Read the model definition and answer for the solid it produces. Units are mm, in the model's axes. Face numbers are marked on the shaded views. A direction names the side the tool comes from. Coordinates: 2 decimals unless noted, no trailing zeros. Order: outer loops, then holes, each group sorted by start corner. A loop starts at its lowest first (then second) coordinate and runs counter-clockwise, first axis right, second up.
from build123d import *

# Parameters (mm, degrees)
R_VOLUTION1_ANGLE  = 180
COQUE1_T           = -2
ESQUISSE2_W        = 60
ESQUISSE2_H        = 8
BOSS_EXTRU_1_DEPTH = 8
CHANFREIN1_SIZE    = 1


with BuildPart() as part:
    # Esquisse1 → Révolution1 (revolve)
    with BuildSketch(Plane.XY):
        with BuildLine():
            Line((-25, 0), (25, 0))
            ThreePointArc((25, 0), (0, 25), (-25, 0))
        make_face()
    revolve(axis=Axis((-25, 0, 0), (1, 0, 0)), revolution_arc=R_VOLUTION1_ANGLE)

    # Coque1
    coque1_openings = [part.faces().sort_by_distance(p)[0] for p in [
        (-25, 0, 0),
    ]]
    offset(amount=COQUE1_T, openings=coque1_openings)

    # Esquisse2 → Boss.-Extru.1 (add)
    with BuildSketch(Plane.XY):
        with Locations((52.649503306, 0)):
            Rectangle(ESQUISSE2_W, ESQUISSE2_H)
    extrude(amount=BOSS_EXTRU_1_DEPTH)

    # Chanfrein1
    chanfrein1_edges = [part.edges().sort_by_distance(p)[0] for p in [
        (82.649503306, -4, 4),
        (82.649503306, 4, 4),
    ]]
    chamfer(chanfrein1_edges, length=CHANFREIN1_SIZE)


solid = part.part
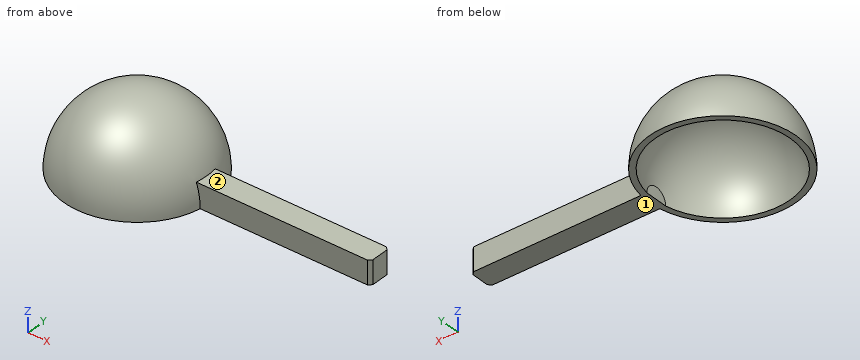
Q1. Which of the six approach directions +Z, -Z, +X, -X, +Y, -Y give full straight-line access (tool end or side, diameter ignored) to the marked faces 1 and 2?
Q2. Each of these flat-tipped pins is pushed along its axis until it touches: P1, Ø4, axis at x = 55.5, z = 2, coming from the +Y side; P2, Ø2, axis at y = 1.5, z = 3, coming from the -X side; P3, Ø12, axis at x = 15.5, y = -16.5, coming from the +Z side; P4, Ø8, axis at y = -1.5, z = 8.5, coming from the +X side. Where does it stop, or does it pass through?
Q3. Straight lines are drawn through the part: L1, parallel to Y at x = 16.5, z = 3; L2, parallel to X at y = -15, z = 9; L3, parallel to X at y = 17, z = 12.75. For each, find the intervals that lie inside material, in ascending order.
Q4. The part is cut by section B-B, the plane x = 32. Determine the outline of the cut face in (y, z), then the cut area to 3 significant figures.
Q5. The part is cut by section A-A, the plane z = 2.25. Determine the outline of the cut face in (x, y), then the cut area to 3 significant figures.
Q6. The part is cut by section D-D, the plane y = -12.5. Determine the outline of the cut face in (x, z), then the cut area to 3 significant figures.
Q7. The part is cut by section C-C, the plane z = 7. Determine the outline of the cut face in (x, y).
Computed values:
1. face 1: -Z, +X, -X, +Y, -Y
1. face 2: +Z, +X, +Y, -Y
2. P1: stops at y = 4
2. P2: stops at x = -24.89
2. P3: stops at z = 18.66
2. P4: stops at x = 82.65
3. L1: y = -18.54 to -15.74, 15.74 to 18.54
3. L2: x = -17.86 to -14.93, 14.93 to 17.86
3. L3: x = -13.17 to -8.8, 8.8 to 13.17
4. outline: (-4, 0) - (4, 0) - (4, 8) - (-4, 8) - close
4. area: 64.0 mm2
5. outline: (24.58, -4) - (81.65, -4) - (82.65, -3) - (82.65, 3) - (81.65, 4) - (24.58, 4) arc R24.9 ccw (long way) to start; hole (22.65, -3.31) - (22.65, 3.31) arc R22.89 ccw (long way) to start
5. area: 765 mm2
6. outline: (-21.65, 0) - (-19.31, 0) arc R19.31 cw to (19.31, 0) - (21.65, 0) arc R21.65 ccw to start
6. area: 151 mm2
7. outline: (23.66, -4) - (81.65, -4) - (82.65, -3) - (82.65, 3) - (81.65, 4) - (23.66, 4) arc R24 ccw (long way) to start; hole circle Ø43.82 at (0, 0)
